Can you work these out from the model? Positions are in its coordinate system, mm. Face numbers are marked on the shaded views. A direction names the side the tool comes from. Give positions to 0.01 mm unless a question says otherwise; leave off trailing zeros. Write each loop counter-clockwise with the first axis right and the second up, starting at its lowest first coordinate (ties: lowest second). Pieces come first, ordered by that corner, then holes. Notation, with made-up numbers: (-2, -9) -> (46, -9) arc R22 cw to (46, 16) -> close; hole circle Ø11 at (52, 16.25). An arc over 180 degrees is marked (long way). One line per item, written item: value.
Autodesk Inventor part; units mm, degrees
ref_plane "YZ Plane" through (0, 0, 0) normal (1, 0, 0) x (0, 1, 0)
ref_plane "XZ Plane" through (0, 0, 0) normal (0, 1, 0) x (-1, 0, 0)
ref_plane "XY Plane" through (0, 0, 0) normal (0, 0, 1) x (1, 0, 0)
sketch "Sketch1" plane through (0, 0, 0) normal (0, 1, 0) x (-1, 0, 0)
  line L0 (2.728, 3.799) -> (-60.772, 3.799)
  line L1 (-60.772, 3.799) -> (-60.772, -47.001)
  line L2 (-60.772, -47.001) -> (2.728, -47.001)
  line L3 (2.728, -47.001) -> (2.728, 3.799)
  dimension "d0" = 63.5
  dimension "d1" = 50.8
extrude "Extrusion1" add sketch "Sketch1" along normal blind 1.5875
sketch "Sketch2" plane through (0, 1.5875, 0) normal (0, 1, 0) x (1, 0, 0)
  line L0 (59.1845, 45.4135) -> (-1.1405, 45.4135)
  line L1 (-1.1405, 45.4135) -> (-1.1405, -2.2115)
  line L2 (-1.1405, -2.2115) -> (59.1845, -2.2115)
  line L3 (59.1845, -2.2115) -> (59.1845, 45.4135)
  line L4 (60.772, 47.001) -> (-2.728, 47.001)
  line L5 (-2.728, 47.001) -> (-2.728, -3.799)
  line L6 (60.772, -3.799) -> (60.772, 47.001)
  line L7 (-2.728, -3.799) -> (60.772, -3.799)
  point P0 (0, 0)
  dimension "d4" = 1.5875
  dimension "d5" = 1.5875
  dimension "d6" = 1.5875
  dimension "d7" = 1.5875
extrude "Extrusion2" add sketch "Sketch2" along normal blind 17.4625
fillet "Fillet1" radius 3.302 8 edges at (29.022, 0, 3.799) (60.772, 0, -21.601) (29.022, 0, -47.001) (-2.728, 0, -21.601) (60.772, 9.525, -47.001) (60.772, 9.525, 3.799) (-2.728, 9.525, 3.799) (-2.728, 9.525, -47.001)
fillet "Fillet2" radius 1.5875 8 edges at (-1.1405, 10.3188, -45.4135) (29.022, 1.5875, -45.4135) (-1.1405, 1.5875, -21.601) (-1.1405, 10.3188, 2.2115) (29.022, 1.5875, 2.2115) (59.1845, 10.3188, 2.2115) (59.1845, 1.5875, -21.601) (59.1845, 10.3188, -45.4135)
sketch "Sketch4" plane through (0, 19.05, 0) normal (0, 1, 0) x (1, 0, 0)
  line L0 (0.447, 45.4135) -> (57.597, 45.4135)
  arc A0 (0.447, 45.4135) -> (-1.1405, 43.826) centre (0.447, 43.826) ccw
  line L1 (-1.1405, -0.624) -> (-1.1405, 43.826)
  arc A1 (59.1845, 43.826) -> (57.597, 45.4135) centre (57.597, 43.826) ccw
  line L2 (59.1845, 43.826) -> (59.1845, -0.624)
  arc A2 (57.597, -2.2115) -> (59.1845, -0.624) centre (57.597, -0.624) ccw
  line L3 (57.597, -2.2115) -> (0.447, -2.2115)
  arc A3 (-1.1405, -0.624) -> (0.447, -2.2115) centre (0.447, -0.624) ccw
  line L4 (0.2977, 46.0073) -> (57.7462, 46.0073)
  line L5 (59.7782, 43.9753) -> (59.7782, -0.7732)
  line L6 (57.7462, -2.8052) -> (0.2977, -2.8052)
  line L7 (-1.7343, -0.7732) -> (-1.7343, 43.9753)
  line L8 (57.47, 47.001) -> (0.574, 47.001)
  line L9 (-2.728, 43.699) -> (-2.728, -0.497)
  arc A4 (0.574, 47.001) -> (-2.728, 43.699) centre (0.574, 43.699) ccw
  arc A5 (60.772, 43.699) -> (57.47, 47.001) centre (57.47, 43.699) ccw
  line L10 (60.772, -0.497) -> (60.772, 43.699)
  arc A6 (57.47, -3.799) -> (60.772, -0.497) centre (57.47, -0.497) ccw
  line L11 (0.574, -3.799) -> (57.47, -3.799)
  arc A7 (-2.728, -0.497) -> (0.574, -3.799) centre (0.574, -0.497) ccw
  line L12 (9.3601, 46.0073) -> (9.3601, 47.001)
  line L13 (9.9735, 46.0073) -> (9.9735, 45.2135)
  line L14 (-1.7343, 35.9118) -> (-2.728, 35.9118)
  line L15 (-1.7343, 35.9118) -> (-1.1405, 35.9118)
  line L16 (3.5402, -2.2115) -> (3.5402, -2.8052)
  line L17 (3.9514, -2.8052) -> (3.9514, -3.799)
  line L18 (59.1845, 4.7048) -> (59.7782, 4.7048)
  line L19 (59.7782, 4.7048) -> (60.772, 4.7048)
  arc A8 (0.2977, 46.0073) -> (-1.7343, 43.9753) centre (0.2977, 43.9753) ccw
  arc A9 (59.7782, 43.9753) -> (57.7462, 46.0073) centre (57.7462, 43.9753) ccw
  arc A10 (-1.7343, -0.7732) -> (0.2977, -2.8052) centre (0.2977, -0.7732) ccw
  arc A11 (57.7462, -2.8052) -> (59.7782, -0.7732) centre (57.7462, -0.7732) ccw
  point P0 (0, 0)
  dimension "d20" = 2.032
  dimension "d21" = 2.032
  dimension "d22" = 2.032
  dimension "d23" = 2.032
  dimension "d26" = 0.9938
  dimension "d27" = 0.9938
  dimension "d28" = 0.9938
  dimension "d29" = 0.9938
extrude "Extrusion4" cut sketch "Sketch4" against normal blind 1.5875 contours L4 L12 L8 A5 L10 L19 L5 A9 | L4 A8 L7 L14 L9 A4 L8 L12 | L7 A10 L6 L17 L11 A7 L9 L14 | L19 L10 A6 L11 L17 L6 A11 L5
ref_plane "Work Plane1" through (-1.1405, 3.175, -33.5073) normal (0.7071, 0.7071, 0) x (0, 0, 1)
sketch "Sketch8" plane through (-1.1405, 3.175, -33.5073) normal (0.7071, 0.7071, 0) x (0, 0, 1)
  line L0 (34.1313, 0) -> (34.1313, 2.2451)
  line L1 (-10.3187, 0) -> (34.1313, 0)
  line L2 (34.1313, 2.2451) -> (-10.3187, 2.2451)
  line L3 (-10.3187, 2.2451) -> (-10.3187, 0)
  line L4 (14.9063, -0.1275) -> (8.9063, -0.1275)
  line L5 (8.9063, -0.1275) -> (8.9063, 2.3725)
  line L6 (8.9063, 2.3725) -> (14.9063, 2.3725)
  line L7 (14.9063, 2.3725) -> (14.9063, -0.1275)
  line L8 (14.9063, 1.1225) -> (34.1313, 1.1225)
  line L9 (8.9063, 1.8195) -> (-10.3187, 1.8195)
  line L10 (14.1632, 0) -> (14.1632, -0.1275)
  line L11 (13.7933, 2.3725) -> (13.7933, 2.2451)
  point P0 (33.5073, 3.0515)
  dimension "d43" = 6
  dimension "d44" = 2.5
extrude "Extrusion7" cut sketch "Sketch8" against normal blind 1.4 contours L7 L4 L10 L1 | L1 L5 L2 L7 | L10 L4 L5 L1 | L2 L11 L6 L7 | L2 L5 L6 L11
ref_plane "Work Plane2" through (-2.728, 3.302, -34.301) normal (1, 0, 0) x (0, 0, -1)
sketch "Sketch9" plane through (-2.728, 3.302, -34.301) normal (1, 0, 0) x (0, 0, -1)
  line L0 (-34.798, 14.1605) -> (9.398, 14.1605)
  line L1 (12.7, 14.1605) -> (12.7, 0)
  line L2 (-38.1, 0) -> (-38.1, 14.1605)
  circle A0 centre (-12.7, 14.1605) radius 3
  line L3 (-12.7, 14.1605) -> (12.7, 14.1605)
  line L4 (12.7, 0) -> (12.7, 14.1605)
  line L5 (-12.7, 14.1605) -> (-38.1, 14.1605)
  line L6 (-38.1, 14.1605) -> (-38.1, 0)
  line L7 (9.398, 14.1605) -> (-34.798, 14.1605)
  line L8 (-9.7, 14.1605) -> (-9.7, 15.748)
  line L9 (-34.925, 15.748) -> (9.525, 15.748)
  line L10 (-15.7, 14.1605) -> (-15.7, 15.748)
  point P0 (-34.301, -3.302)
  dimension "d47" = 6
extrude "Extrusion9" cut sketch "Sketch9" along normal blind 3
equation "\"d5\" = d4"
equation "\"d6\" = d4"
equation "\"d7\" = d4"
properties part number "RFID_Box"
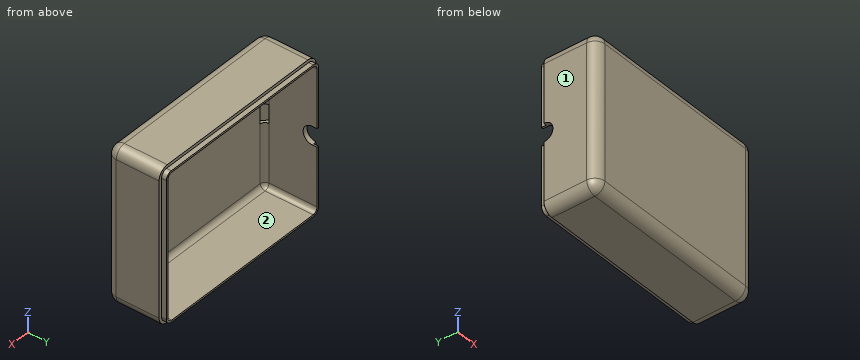
1) If we section it at D-D (y = 16): Write out the boundary of the cut face in (x, z) (1 decimal), and give its area (3 significant figures).
Answer list:
outline: (-2.7, -43.7) arc R3.3 ccw to (0.6, -47) -> (57.5, -47) arc R3.3 ccw to (60.8, -43.7) -> (60.8, 0.5) arc R3.3 ccw to (57.5, 3.8) -> (0.6, 3.8) arc R3.3 ccw to (-2.7, 0.5) -> (-2.7, -19) -> (-1.1, -19) -> (-1.1, 0.6) arc R1.6 cw to (0.4, 2.2) -> (57.6, 2.2) arc R1.6 cw to (59.2, 0.6) -> (59.2, -43.8) arc R1.6 cw to (57.6, -45.4) -> (0.4, -45.4) arc R1.6 cw to (-1.1, -43.8) -> (-1.1, -24.2) -> (-2.7, -24.2) -> close
area: 337 mm^2
2) I need wall thicknesses on L1, parallel to Z at x = 43, y = 8.75; L2, parallel to X at y = 15.5, z = -43; L3, parallel to Z at x = 51.5, y = 18. Which ranges of each line are inside material? Lowest first, please.
Answer list:
L1: z = -47 to -45.41, 2.21 to 3.8
L2: x = -2.73 to -1.14, 59.18 to 60.77
L3: z = -46.01 to -45.41, 2.21 to 2.81
3) For the marked faces 1 and 2, which set-ups out of +Z, -Z, +X, -X, +Y, -Y let a thin tool reach every point of the face, with its end or its side?
Answer list:
face 1: +Z, -Z, -X, +Y, -Y
face 2: +Y
4) Will these pins go through, and if not, where does the flat tip stop? pin 1 (1 mm diameter, centred on x = 29, z = -32, fed in from -Y); pin 2 (0.8 mm diameter, centred on x = 17.5, y = 18.5, fed in from -Z); pin 3 (6 mm diameter, centred on x = 15, z = -42, fed in from +Y); pin 4 (1.4 mm diameter, centred on x = -0.5, y = 2, fed in from -Z).
Answer list:
pin 1: stops at y = 0
pin 2: stops at z = -46.01
pin 3: stops at y = 2.11
pin 4: stops at z = -46.85
5) If we section it at A-A (y = 12): Write out the boundary of the cut face in (x, z) (1 decimal).
Answer list:
outline: (-2.7, -43.7) arc R3.3 ccw to (0.6, -47) -> (57.5, -47) arc R3.3 ccw to (60.8, -43.7) -> (60.8, 0.5) arc R3.3 ccw to (57.5, 3.8) -> (0.6, 3.8) arc R3.3 ccw to (-2.7, 0.5) -> close; hole (-1.1, -43.8) arc R1.6 ccw to (0.4, -45.4) -> (57.6, -45.4) arc R1.6 ccw to (59.2, -43.8) -> (59.2, 0.6) arc R1.6 ccw to (57.6, 2.2) -> (0.4, 2.2) arc R1.6 ccw to (-1.1, 0.6) -> close
